The model under review builds one solid part; all positions refer to its coordinate system, in mm. Face numbers are marked on the shaded views. A direction names the side the tool comes from. Coordinates: 2 decimals unless noted, no trailing zeros. Loops run counter-clockwise (first coordinate to the right, second up) from the corner with the lowest first, then second, coordinate; pieces in that order, holes last. Notation, with made-up numbers: M -31.75,73.25 L 12.25,73.25 A23 ccw 12.25,97.25 Z; hole C 70,4.25 d9. An arc over 180 degrees is marked long. Write item = value, one per line. Start each with the question number.
Q1. We need section A-A on y = 3. Give the boundary of the cut face in (x, z), and give its area (3 significant figures).
Q2. Mouldability with a two-part tool opening along X and no side actions: class the marked faces 4, 5 and 6 as released by +X, released by -X, zero draft, split by the parting line, or undercut.
Q3. Clearance check with flat-ended pins moving along their axes: pin 1 Ø12 at (x, z) = (7, -2) entering from +Y; pin 2 Ø1.5 at (x, y) = (15.5, 11) entering from +Z; pin 3 Ø5 at (x, y) = (16, 13.5) entering from -Z; pin 4 Ø8 at (x, y) = (-2, 9.5) entering from -Z. State where each tip first meets the part, or that it passes through.
Q4. We need section D-D on x = 9. Give the boundary of the cut face in (y, z), and give its area (3 significant figures).
Q5. For the marked faces 1, 2 and 3, list the 3-axis set-ups (+Z, -Z, +X, -X, +Y, -Y) from which the entire face can be reached by the end or side of a thin tool; tool diameter is ignored.
Q6. We need section B-B on x = -0.5. Give the boundary of the cut face in (y, z).
Q7. Wall thickness on probe 1 along Y at (x, z) = (0, 7); probe 2 along Z at (x, y) = (2, 2.25); probe 3 along Z at (x, y) = (2.75, 11.25): over which ranges is each line inside the solid? List them lowest first.
Q8. We need section C-C on z = -10.75. Give the boundary of the cut face in (x, y).
from build123d import *

# Parameters (mm, degrees)
SALIENTE_EXTRUIR1_DEPTH = 15
VACIADO1_T              = -0.5


with BuildPart() as part:
    # Croquis2 → Saliente-Extruir1 (new body)
    with BuildSketch(Plane(origin=(0, 0, 0), x_dir=(1, 0, 0), z_dir=(0, 1, 0))):
        Polygon((20, 0), (-6.05, 13.239344826), (0, 0), (-6.05, -13.239344826), align=None)
    extrude(amount=SALIENTE_EXTRUIR1_DEPTH)

    # Vaciado1
    vaciado1_openings = [part.faces().sort_by_distance(p)[0] for p in [
        (4.65, 15, 0),
    ]]
    offset(amount=VACIADO1_T, openings=vaciado1_openings, kind=Kind.INTERSECTION)


solid = part.part
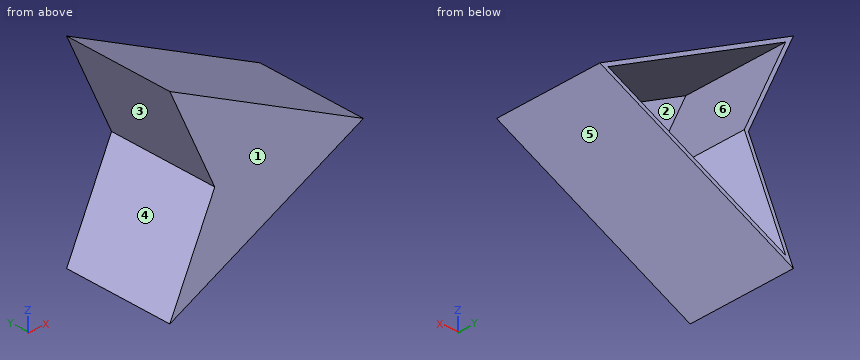
Returned:
q1.outline = M -6.05,-13.24 L 20,0 L -6.05,13.24 L 0,0 Z; hole M -5,-12.14 L 18.9,0 L -5,12.14 L 0.55,0 Z
q1.area = 42.0 mm^2
q2.face_4 = released by -X
q2.face_5 = released by +X
q2.face_6 = undercut
q3.pin_1 = 15
q3.pin_2 = 2.67
q3.pin_3 = -3.3
q3.pin_4 = -13.21
q4.outline = M 0,-5.59 L 15,-5.59 L 15,-5.03 L 0.5,-5.03 L 0.5,5.03 L 15,5.03 L 15,5.59 L 0,5.59 Z
q4.area = 21.9 mm^2
q5.face_1 = +Z, -Z, +X, -X, -Y
q5.face_2 = +Y
q5.face_3 = -X, +Y, -Y
q6.outline = M 0,-10.42 L 15,-10.42 L 15,-9.86 L 0.5,-9.86 L 0.5,-2.3 L 15,-2.3 L 15,-1.09 L 0,-1.09 Z; M 0,1.09 L 15,1.09 L 15,2.3 L 0.5,2.3 L 0.5,9.86 L 15,9.86 L 15,10.42 L 0,10.42 Z
q7.probe_1 = 0 to 0.5
q7.probe_2 = -9.15 to -8.59, 8.59 to 9.15
q7.probe_3 = -8.77 to -8.21, 8.21 to 8.77
q8.outline = M -4.91,0 L -1.15,0 L -1.15,15 L -2.26,15 L -2.26,0.5 L -4.36,0.5 L -4.36,15 L -4.91,15 Z
